from build123d import *

# Parameters (mm, degrees)
SKETCH1_W                = 15
SKETCH1_H                = 35
SKETCH1_R                = 1.5
BOSS_EXTRUDE1_DEPTH      = 1.5
SKETCH2_R                = 5
BOSS_EXTRUDE2_DEPTH      = 2
BOSS_EXTRUDE2_DEPTH_BACK = 4
SKETCH3_R                = 4
CUT_EXTRUDE1_DEPTH       = 0.1
SKETCH4_W                = 4
SKETCH4_H                = 10
BOSS_EXTRUDE3_DEPTH      = 10


with BuildPart() as part:
    # Sketch1 → Boss-Extrude1 (new body)
    with BuildSketch(Plane.XY):
        with Locations((220.135234982, 151.894136477)):
            Rectangle(SKETCH1_W, SKETCH1_H)
        with Locations((220.135234982, 143.394136477)):
            Circle(SKETCH1_R, mode=Mode.SUBTRACT)
    extrude(amount=BOSS_EXTRUDE1_DEPTH)

    # Sketch2 → Boss-Extrude2 (add, two sides)
    with BuildSketch(Plane(origin=(0, 169.394136477, 0), x_dir=(1, 0, 0), z_dir=(0, 1, 0))) as boss_extrude2_sk:
        with Locations((220.135234982, 3.1)):
            Circle(SKETCH2_R)
    extrude(amount=BOSS_EXTRUDE2_DEPTH)
    extrude(boss_extrude2_sk.sketch, amount=-BOSS_EXTRUDE2_DEPTH_BACK)

    # Sketch3 → Cut-Extrude1 (cut)
    with BuildSketch(Plane(origin=(0, 171.394136477, 0), x_dir=(1, 0, 0), z_dir=(0, 1, 0))):
        with Locations((220.135234982, 3.1)):
            Circle(SKETCH3_R)
    extrude(amount=-CUT_EXTRUDE1_DEPTH, mode=Mode.SUBTRACT)

    # Sketch4 → Boss-Extrude3 (add)
    with BuildSketch(Plane(origin=(0, 0, 0), x_dir=(-1, 0, 0), z_dir=(0, 0, -1))):
        with Locations((-225.135234982, 153.394136477)):
            Rectangle(SKETCH4_W, SKETCH4_H)
    extrude(amount=BOSS_EXTRUDE3_DEPTH)


solid = part.part
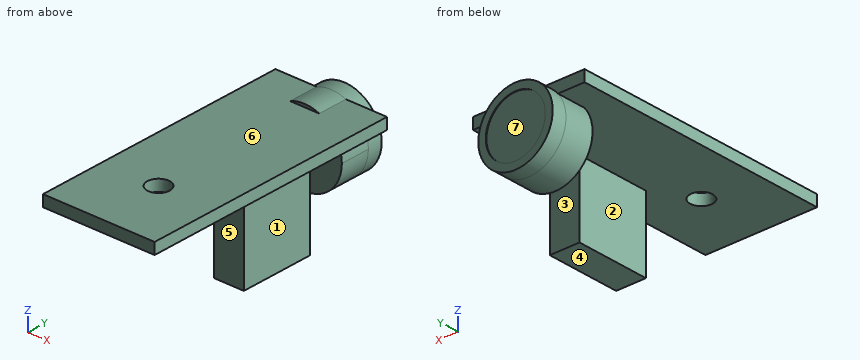
Read the model definition and answer for the solid it produces. Units are mm, in the model's axes. Face numbers are marked on the shaded views. A direction names the side the tool comes from. Round coordinates to 2 decimals unless told otherwise and drop trailing zeros. Loops run counter-clockwise (first coordinate to the right, second up) from the corner with the lowest first, then second, coordinate; pieces in that order, holes last. Notation, with made-up numbers: (64, 28.5) - (113, 28.5) arc R17 ccw to (113, 54.5) - close; hole circle Ø4 at (-27.75, 26). An arc over 180 degrees is marked (long way). One line per question, with ' | ' between items. Start each with the question number.
Q1. Section D-D on y = 153 is taken. Give the vertices of the cut face in (x, z).
Q2. Find the intervals of material crossed by L1, parallel to X at y = 171.35, z = -3.1; L2, parallel to Y at x = 223.5, z = -5.5; L3, parallel to X at y = 152, z = -6.25, in increasing order.
Q3. For a pull along Z with two mould halves and no side action, classify the marked faces 4, 5, 6 and 7 as +Z half, -Z half, draft (parallel to the pull), parting line (faces both ways), or undercut.
Q4. Section B-B on x = 219.25 is taken. Give the vertices of the cut face in (y, z).
Q5. Section A-A on z = -4.25 is taken. Give the vertices of the cut face in (x, y), plus the area to 3 significant figures.
Q6. For the marked faces 1, 2 and 3, determine the directions among +Z, -Z, +X, -X, +Y, -Y from which every point of the face is accessible in a straight line to the end or side of a thin tool.
Q7. Flat-ended cylindrical pins translate along their axes: pin 1 (4.5 mm diameter, centred on x = 216.5, y = 153.5, fed in from +Z); pin 2 (3 mm diameter, centred on y = 152.5, z = -5.5, fed in from +X); pin 3 (1.2 mm diameter, centred on x = 215, z = 1, fed in from +Y). Find the tip coordinate at first contact, or state that the pin passes through.
Q8. Section C-C on y = 143 is taken. Give the vertices of the cut face in (x, z), plus the area to 3 significant figures.
Established:
1) outline: (212.64, 0) - (223.14, 0) - (223.14, -10) - (227.14, -10) - (227.14, 0) - (227.64, 0) - (227.64, 1.5) - (212.64, 1.5) - close
2) L1: 215.14 to 216.14, 224.14 to 225.14 | L2: 148.39 to 158.39, 165.39 to 171.39 | L3: 223.14 to 227.14
3) face 4: -Z half | face 5: draft | face 6: +Z half | face 7: undercut
4) outline: (134.39, 0) - (142.18, 0) - (142.18, 1.5) - (134.39, 1.5) - close; (144.61, 0) - (165.39, 0) - (165.39, -8.02) - (171.39, -8.02) - (171.39, -7) - (171.29, -7) - (171.29, 0.8) - (171.39, 0.8) - (171.39, 1.82) - (165.39, 1.82) - (165.39, 1.5) - (144.61, 1.5) - close
5) outline: (215.27, 165.39) - (225, 165.39) - (225, 171.39) - (223.97, 171.39) - (223.97, 171.29) - (216.3, 171.29) - (216.3, 171.39) - (215.27, 171.39) - close; (223.14, 148.39) - (227.14, 148.39) - (227.14, 158.39) - (223.14, 158.39) - close | area: 97.6 mm²
6) face 1: -Z, +X, +Y, -Y | face 2: -Z, -X, -Y | face 3: -Z, +X, -X
7) pin 1: z = 1.5 | pin 2: x = 227.14 | pin 3: y = 169.39
8) outline: (212.64, 0) - (218.69, 0) - (218.69, 1.5) - (212.64, 1.5) - close; (221.58, 0) - (227.64, 0) - (227.64, 1.5) - (221.58, 1.5) - close | area: 18.2 mm²
